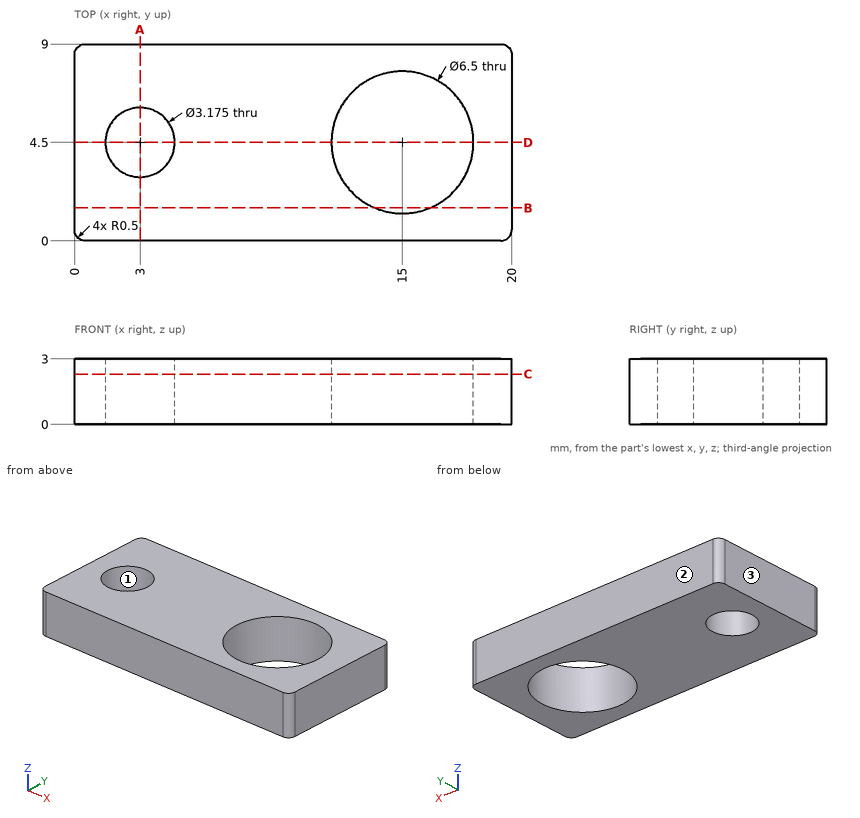
The figure shows three views and two pictorial views of one solid part (mm, origin at its lowest corner). Answer the questions. Give positions to 0.01 mm unless a question says otherwise; leave off trailing zeros. Order: outer loops, then holes, each group sorted by start corner. A loop starts at its lowest first (then second) coordinate and runs counter-clockwise, first axis right, second up. Notation, with made-up numbers: M 17.25,-22.5 L 63.25,-22.5 A18 ccw 63.25,11.5 Z; hole C 73.5,-25 d10. An arc over 180 degrees is marked long. Return JSON: item names as keys, results as strings.
1) Section A-A, the plane x = 3 is taken. Write down the section's boundary in (y, z).
Resolved:
{"outline": "M 0,0 L 2.91,0 L 2.91,3 L 0,3 Z; M 6.09,0 L 9,0 L 9,3 L 6.09,3 Z"}
2) Straight lines are drawn through the part: line 1 along Y through (x, z) = (3, 0.8); line 2 along Y through (x, z) = (15, 0.8); line 3 along X through (y, z) = (5.5, 1). For each, find the intervals that lie inside material, in ascending order. Write a range as [from, to].
Resolved:
{"line 1": "[0, 2.91], [6.09, 9]", "line 2": "[0, 1.25], [7.75, 9]", "line 3": "[0, 1.77], [4.23, 11.91], [18.09, 20]"}
3) For a pull along Y with two mould halves and no side action, classify the marked faces 1, 2 and 3 as +Y half, -Y half, draft (parallel to the pull), parting line (faces both ways), or undercut.
Resolved:
{"face 1": "undercut", "face 2": "+Y half", "face 3": "draft"}
4) Section D-D, the plane y = 4.5 is taken. Write down the section's boundary in (x, z), plus the area to 3 significant figures.
Resolved:
{"outline": "M 0,0 L 1.41,0 L 1.41,3 L 0,3 Z; M 4.59,0 L 11.75,0 L 11.75,3 L 4.59,3 Z; M 18.25,0 L 20,0 L 20,3 L 18.25,3 Z", "area": "31.0 mm^2"}
5) Section C-C, the plane z = 2.3 is taken. Give the number of separate pieces and of enclosed holes in the cut face, plus the area to 3 significant figures.
Resolved:
{"separate pieces": "1", "enclosed holes": "2", "area": "139 mm^2"}
6) Section B-B, the plane y = 1.5 is taken. Write down the section's boundary in (x, z).
Resolved:
{"outline": "M 0,0 L 13.75,0 L 13.75,3 L 0,3 Z; M 16.25,0 L 20,0 L 20,3 L 16.25,3 Z"}
